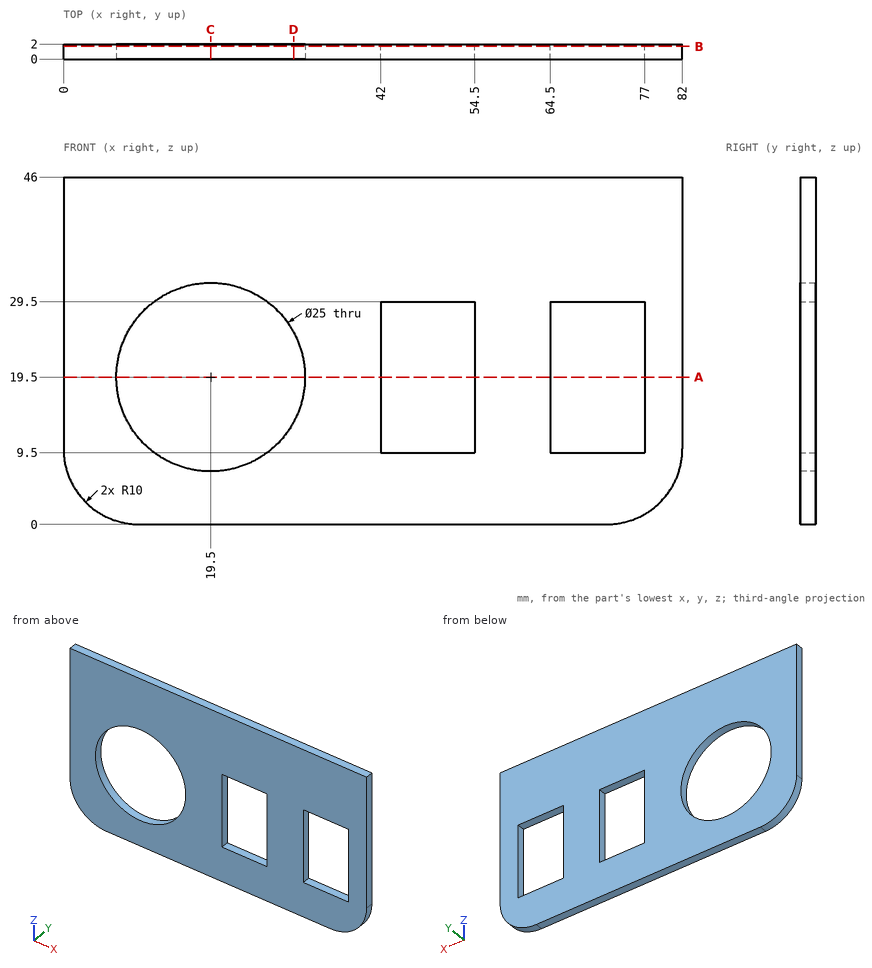
Part print with two shaded views. Sizes in mm from the minimum x, y, z corner. Round coordinates to 2 decimals unless told otherwise and drop trailing zeros. Order: outer loops, then holes, each group sorted by start corner. A loop starts at its lowest first (then second) coordinate and runs counter-clockwise, first axis right, second up.
(1) Band-saw the part on D-D (x = 30.5). List the corners of the cut face in (y, z), then the cut area to 3 significant figures.
(2) Band-saw the part on A-A (z = 19.5). List the corners of the cut face in (x, y).
(3) Drill centre lines: line 1 (X direction, y = 1.1, z = 19.5); line 2 (Z direction, x = 65, y = 0.95); line 3 (X direction, y = 0.65, z = 26.5). Where is each one in solid material? Low to high.
(4) Band-saw the part on B-B (y = 1.7). List the corners of the cut face in (x, z), then the cut area to 3 significant figures.
(5) Band-saw the part on C-C (x = 19.5). List the corners of the cut face in (y, z).
Verdict:
1. outline: (0, 0) - (2, 0) - (2, 13.56) - (0, 13.56) - close; (0, 25.44) - (2, 25.44) - (2, 46) - (0, 46) - close
1. area: 68.3 mm2
2. outline: (0, 0) - (7, 0) - (7, 2) - (0, 2) - close; (32, 0) - (42, 0) - (42, 2) - (32, 2) - close; (54.5, 0) - (64.5, 0) - (64.5, 2) - (54.5, 2) - close; (77, 0) - (82, 0) - (82, 2) - (77, 2) - close
3. line 1: x = 0 to 7, 32 to 42, 54.5 to 64.5, 77 to 82
3. line 2: z = 0 to 9.5, 29.5 to 46
3. line 3: x = 0 to 9.14, 29.86 to 42, 54.5 to 64.5, 77 to 82
4. outline: (0, 10) arc R10 ccw to (10, 0) - (72, 0) arc R10 ccw to (82, 10) - (82, 46) - (0, 46) - close; hole circle Ø25 at (19.5, 19.5); hole (42, 9.5) - (54.5, 9.5) - (54.5, 29.5) - (42, 29.5) - close; hole (64.5, 9.5) - (77, 9.5) - (77, 29.5) - (64.5, 29.5) - close
4. area: 2,740 mm2
5. outline: (0, 0) - (2, 0) - (2, 7) - (0, 7) - close; (0, 32) - (2, 32) - (2, 46) - (0, 46) - close
